Autodesk Inventor part; units mm, degrees
ref_plane "YZ Plane" through (0, 0, 0) normal (1, 0, 0) x (0, 1, 0)
ref_plane "XZ Plane" through (0, 0, 0) normal (0, 1, 0) x (-1, 0, 0)
ref_plane "XY Plane" through (0, 0, 0) normal (0, 0, 1) x (1, 0, 0)
sketch "Sketch1" plane through (0, 0, 0) normal (0, 1, 0) x (-1, 0, 0)
  line L0 (0, 0) -> (-6.35, 0)
  line L1 (-6.35, 0) -> (-6.35, -76.2)
  line L2 (-6.35, -76.2) -> (0, -76.2)
  line L3 (0, -76.2) -> (0, 0)
  line L4 (-6.35, -72.8797) -> (-161.925, -180.975)
  line L5 (-158.3017, -186.1898) -> (0, -76.2)
  line L6 (-158.3017, -186.1898) -> (-161.925, -180.975)
  point P0 (-6.35, -38.1)
  point P1 (-3.175, -76.2)
  point P2 (-6.35, -6.35)
  dimension "d9" = 6.35
  dimension "d10" = 76.2
  dimension "d30" = 6.35
  dimension "d31" = 6.35
  dimension "d32" = 155.575
  dimension "d33" = 174.625
  dimension "d53" = 6.35
extrude "Extrusion1" add sketch "Sketch1" along normal blind 76.2
sketch "Sketch2" plane through (0, 0, -76.2) normal (-1, 0, 0) x (0, 0, 1)
  circle A0 centre (63.5, 12.7) radius 3.2639
  circle A1 centre (63.5, 38.1) radius 3.2639
  circle A2 centre (63.5, 63.5) radius 3.2639
  line L0 (0, 0) -> (0, 76.2)
  line L1 (0, 0) -> (76.2, 0)
  line L2 (76.2, 0) -> (76.2, 76.2)
  circle A3 centre (38.1, 63.5) radius 3.2639
  circle A4 centre (38.1, 38.1) radius 3.2639
  circle A5 centre (38.1, 12.7) radius 3.2639
  dimension "d18" = 6.5278
  dimension "d19" = 25.4
  dimension "d21" = 25.4
  dimension "d22" = 12.7
  dimension "d34" = 12.7
  dimension "d35" = 25.4
  dimension "d36" = 25.4
  dimension "d38" = 25.4
extrude "Extrusion2" cut sketch "Sketch2" against normal through all
sketch "Sketch4" plane through (161.925, 0, -180.975) normal (0.5706, 0, 0.8212) x (0.8212, 0, -0.5706)
  arc A0 (-9.525, 66.675) -> (-15.875, 66.675) centre (-12.7, 66.675) ccw
  arc A1 (-15.875, 60.325) -> (-9.525, 60.325) centre (-12.7, 60.325) ccw
  line L0 (-12.7, 76.4683) -> (-12.7, 0) construction
  line L1 (-189.4417, 0) -> (0, 0) construction
  line L2 (0, 0) -> (0, 76.2) construction
  line L3 (-15.875, 66.675) -> (-15.875, 60.325)
  line L4 (-9.525, 66.675) -> (-9.525, 60.325)
  arc A2 (-9.525, 41.275) -> (-15.875, 41.275) centre (-12.7, 41.275) ccw
  line L5 (-15.875, 41.275) -> (-15.875, 34.925)
  line L6 (-9.525, 41.275) -> (-9.525, 34.925)
  arc A3 (-15.875, 34.925) -> (-9.525, 34.925) centre (-12.7, 34.925) ccw
  arc A4 (-9.525, 15.875) -> (-15.875, 15.875) centre (-12.7, 15.875) ccw
  line L7 (-15.875, 15.875) -> (-15.875, 9.525)
  line L8 (-9.525, 15.875) -> (-9.525, 9.525)
  arc A5 (-15.875, 9.525) -> (-9.525, 9.525) centre (-12.7, 9.525) ccw
  point P0 (-236.2416, 0)
  point P1 (-182.3346, 0)
  point P2 (-9.525, 63.5)
  point P3 (-9.525, 38.1)
  point P4 (-9.525, 12.7)
  dimension "d39" = 6.35
  dimension "d40" = 6.35
  dimension "d41" = 6.35
  dimension "d42" = 12.7
  dimension "d43" = 63.5
  dimension "d46" = 25.4
extrude "Extrusion3" cut sketch "Sketch4" against normal through all
properties part number "INDX_006_Funnel" material "ABS Plastic"
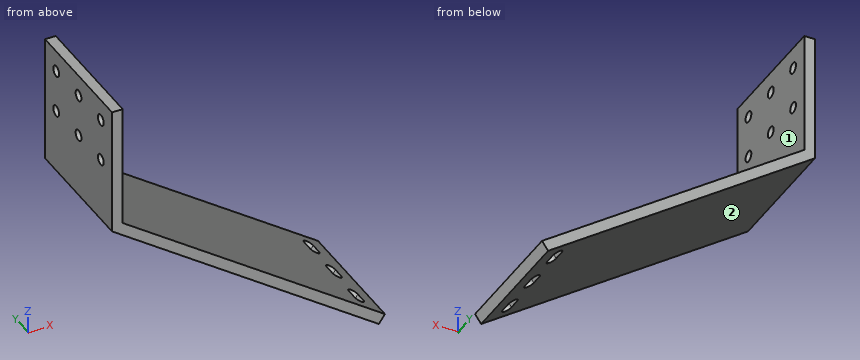
Model file for the job. Use its own axes, mm. Face numbers are marked on the shaded views. A direction names the side the tool comes from. Give positions to 0.01 mm unless a question says otherwise; leave off trailing zeros. Loops run counter-clockwise (first coordinate to the right, second up) from the corner with the lowest first, then second, coordinate; pieces in that order, holes last. Notation, with made-up numbers: (-27.5, 13.5) -> (16.5, 13.5) arc R26 cw to (16.5, 31.5) -> close; hole circle Ø3 at (-21, -36). An arc over 180 degrees is marked (long way). Use CSV: the item, a comma, the result in double quotes. Start each with the question number.
1) Wall check: line 1 (Y direction, x = 4, z = -12); line 2 (Y direction, x = 4, z = -38); line 3 (Z direction, x = 3, y = 38). Give the ranges that are in metal, low to high.
2) Slice it at D-D on z = -54.5. Give the cut face in (x, y), plus the area to 3 significant figures.
3) Slice it at A-A on z = -12.7. Give the cut face in (x, y).
4) Flat gauge pins, fed straight in: pin 1 Ø4 at (y, z) = (11, -156) entering from +X; pin 2 Ø5 at (y, z) = (38.1, -12.7) entering from -X; pin 3 Ø2 at (x, y) = (111, 33.5) entering from -Z; pin 4 Ø6 at (y, z) = (18, -91) entering from -X. Where does each tip first touch, or does it go through?
5) Slice it at B-B on y = 38.1. Give the cut face in (x, z) (3 decimals).
6) Tool access for the marked faces 1 and 2: list every direction of +Z, -Z, +X, -X, +Y, -Y with a clear straight run to the whole face (end or side of a thin tool).
7) Slice it at C-C on y = 26.5. Give the cut face in (x, z) (3 decimals).
Computed values:
1,line 1,"y = 0 to 9.51, 15.89 to 34.91, 41.29 to 60.31, 66.69 to 76.2"
1,line 2,"y = 0 to 9.44, 15.96 to 34.84, 41.36 to 60.24, 66.76 to 76.2"
1,line 3,"z = -78.28 to -41.36, -34.84 to -15.96, -9.44 to 0"
2,outline,"(0, 0) -> (6.35, 0) -> (6.35, 76.2) -> (0, 76.2) -> close"
2,area,"484 mm^2"
3,outline,"(0, 0) -> (6.35, 0) -> (6.35, 9.44) -> (0, 9.44) -> close; (0, 15.96) -> (6.35, 15.96) -> (6.35, 34.84) -> (0, 34.84) -> close; (0, 41.36) -> (6.35, 41.36) -> (6.35, 60.24) -> (0, 60.24) -> close; (0, 66.76) -> (6.35, 66.76) -> (6.35, 76.2) -> (0, 76.2) -> close"
4,pin 1,"stops at x = 128.86"
4,pin 2,"passes through"
4,pin 3,"stops at z = -154.02"
4,pin 4,"stops at x = 16.98"
5,outline,"(0, -76.2) -> (145.265, -177.131) -> (148.888, -171.917) -> (6.35, -72.88) -> (6.35, -41.364) -> (0, -41.364) -> close; (0, -34.836) -> (6.35, -34.836) -> (6.35, -15.964) -> (0, -15.964) -> close; (0, -9.436) -> (6.35, -9.436) -> (6.35, 0) -> (0, 0) -> close; (150.479, -180.755) -> (158.302, -186.19) -> (161.925, -180.975) -> (154.103, -175.54) -> close"
6,face 1,"+Z, +X, +Y, -Y"
6,face 2,"-Z, -X, +Y, -Y"
7,outline,"(0, -76.2) -> (158.302, -186.19) -> (161.925, -180.975) -> (6.35, -72.88) -> (6.35, 0) -> (0, 0) -> close"
